Read the model definition and answer for the solid it produces. Units are mm, in the model's axes. Round coordinates to 2 decimals unless told otherwise and drop trailing zeros. Loops run counter-clockwise (first coordinate to the right, second up) from the corner with the lowest first, then second, coordinate; pieces in that order, holes last. Notation, with made-up numbers: M -32,13.25 L 10,13.25 A10 cw 10,30.25 Z; hole C 31,-36 d10. An arc over 180 degrees is marked long. Answer as CSV lines item,"result".
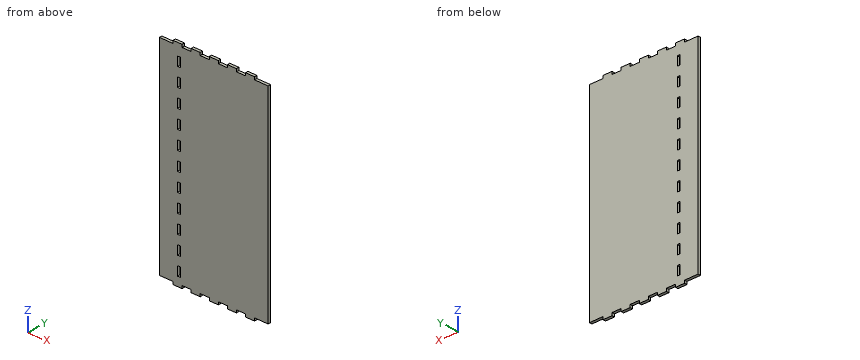
```python
from build123d import *

# Parameters (mm, degrees)
SKETCH1_W           = 120
SKETCH1_H           = 227
BOSS_EXTRUDE1_DEPTH = 3
SKETCH2_W           = 10
SKETCH2_H           = 3
BOSS_EXTRUDE2_DEPTH = 3
LPATTERN1_COUNT     = 5
LPATTERN1_PITCH     = 20
SKETCH3_W           = 10
SKETCH3_H           = 3
BOSS_EXTRUDE3_DEPTH = 3
LPATTERN2_COUNT     = 5
LPATTERN2_PITCH     = 20
SKETCH4_W           = 3
SKETCH4_H           = 10
CUT_EXTRUDE1_DEPTH  = 4
LPATTERN3_COUNT     = 11
LPATTERN3_PITCH     = 20


with BuildPart() as part:
    # Sketch1 → Boss-Extrude1 (new body)
    with BuildSketch(Plane(origin=(0, 0, 0), x_dir=(1, 0, 0), z_dir=(0, 1, 0))):
        with Locations((60, 113.5)):
            Rectangle(SKETCH1_W, SKETCH1_H)
    extrude(amount=BOSS_EXTRUDE1_DEPTH)

    # Sketch2 → Boss-Extrude2 (add)
    with BuildSketch(Plane.XY):
        with Locations((20, 1.5)):
            Rectangle(SKETCH2_W, SKETCH2_H)
    boss_extrude2 = extrude(amount=BOSS_EXTRUDE2_DEPTH)

    # LPattern1: Boss-Extrude2 ×5
    with Locations(*[(i * LPATTERN1_PITCH, 0, 0) for i in range(1, LPATTERN1_COUNT)]):
        add(boss_extrude2)

    # Sketch3 → Boss-Extrude3 (add)
    with BuildSketch(Plane(origin=(0, 0, -227), x_dir=(-1, 0, 0), z_dir=(0, 0, -1))):
        with Locations((-100, 1.5)):
            Rectangle(SKETCH3_W, SKETCH3_H)
    boss_extrude3 = extrude(amount=BOSS_EXTRUDE3_DEPTH)

    # LPattern2: Boss-Extrude3 ×5
    with Locations(*[(-i * LPATTERN2_PITCH, 0, 0) for i in range(1, LPATTERN2_COUNT)]):
        add(boss_extrude3)

    # Sketch4 → Cut-Extrude1 (cut, through all)
    with BuildSketch(Plane(origin=(0, 3, 0), x_dir=(1, 0, 0), z_dir=(0, 1, 0))):
        with Locations((21.5, 15)):
            Rectangle(SKETCH4_W, SKETCH4_H)
    cut_extrude1 = extrude(amount=-CUT_EXTRUDE1_DEPTH, mode=Mode.SUBTRACT)

    # LPattern3: Cut-Extrude1 ×11
    with Locations(*[(0, 0, -i * LPATTERN3_PITCH) for i in range(1, LPATTERN3_COUNT)]):
        add(cut_extrude1, mode=Mode.SUBTRACT)


solid = part.part
```
1) Each of these flat-tipped pins is pushed along its axis until it touches: P1, Ø1.5, axis at y = 2, z = -228.5, coming from the +X side; P2, Ø1.5, axis at x = 94.5, y = 2.5, coming from the +Z side; P3, Ø0.9, axis at y = 1.5, z = -228, coming from the -X side; P4, Ø0.9, axis at x = 115, y = 2, coming from the -Z side. Where does it stop, or does it pass through?
Evaluation:
P1,"stops at x = 105"
P2,"stops at z = 3"
P3,"stops at x = 15"
P4,"stops at z = -227"
2) Straight lines are drawn through the part: line 1 (X direction, y = 2.15, z = -178); line 2 (Z direction, x = 114, y = 2.75). For each, find the intervals that lie inside material, in ascending order.
Evaluation:
line 1,"x = 0 to 20, 23 to 120"
line 2,"z = -227 to 0"
3) Find section B-B, the plane y = 1.4. Count the separate pieces of the cut face and the enclosed holes in it, then the cut area to 3 significant figures.
Evaluation:
separate pieces,"1"
enclosed holes,"11"
area,"27,200 mm^2"
4) Find section A-A, the plane z = -176.5. Give the vertices of the cut face in (x, y), then the cut area to 3 significant figures.
Evaluation:
outline,"M 0,0 L 20,0 L 20,3 L 0,3 Z; M 23,0 L 120,0 L 120,3 L 23,3 Z"
area,"351 mm^2"
5) Find section C-C, the plane x = 68. Give the vertices of the cut face in (y, z), then the cut area to 3 significant figures.
Evaluation:
outline,"M 0,-227 L 3,-227 L 3,0 L 0,0 Z"
area,"681 mm^2"
